Autodesk Inventor part; units mm, degrees
ref_plane "YZ Plane" through (0, 0, 0) normal (1, 0, 0) x (0, 1, 0)
ref_plane "XZ Plane" through (0, 0, 0) normal (0, 1, 0) x (-1, 0, 0)
ref_plane "XY Plane" through (0, 0, 0) normal (0, 0, 1) x (1, 0, 0)
sketch "Sketch1" plane through (0, 0, 0) normal (0, 1, 0) x (-1, 0, 0)
  line L0 (0, 0) -> (-100, 0)
  line L1 (-100, 0) -> (-100, -24.25)
  line L2 (-100, -24.25) -> (-86, -24.25)
  arc A0 (-86, -50.25) -> (-86, -24.25) centre (-86, -37.25) ccw
  line L3 (-86, -50.25) -> (-100, -50.25)
  line L4 (-100, -50.25) -> (-100, -74.5)
  line L5 (-100, -74.5) -> (0, -74.5)
  line L6 (0, -74.5) -> (0, -50.25)
  line L7 (0, -50.25) -> (-14, -50.25)
  arc A1 (-14, -24.25) -> (-14, -50.25) centre (-14, -37.25) ccw
  line L8 (-14, -24.25) -> (0, -24.25)
  line L9 (0, -24.25) -> (0, 0)
  circle A2 centre (-14, -62.25) radius 2.25
  circle A3 centre (-14, -12.25) radius 2.25
  circle A4 centre (-86, -62.25) radius 2.25
  circle A5 centre (-86, -12.25) radius 2.25
  dimension "d0" = 13
  dimension "d1" = 50
  dimension "d2" = 4.5
  dimension "d3" = 25
  dimension "d5" = 12.25
  dimension "d6" = 100
  dimension "d10" = 14
extrude "Extrusion1" add sketch "Sketch1" along normal blind 6.5
sketch "Sketch3" plane through (0, 6.5, 0) normal (0, 1, 0) x (1, 0, 0)
  line L0 (100, 74.5) -> (0, 74.5)
  line L1 (22.75, 74.5) -> (27.25, 74.5)
  line L2 (27.25, 58.2) -> (22.75, 58.2)
  line L3 (29.75, 69.5) -> (29.75, 62.2)
  line L4 (20.25, 62.2) -> (20.25, 69.5)
  line L5 (27.25, 74.5) -> (27.25, 69.5)
  line L6 (27.25, 62.2) -> (27.25, 58.2)
  line L7 (22.75, 58.2) -> (22.75, 62.2)
  line L8 (22.75, 69.5) -> (22.75, 74.5)
  line L9 (20.25, 69.5) -> (22.75, 69.5)
  line L10 (27.25, 69.5) -> (29.75, 69.5)
  line L11 (29.75, 62.2) -> (27.25, 62.2)
  line L12 (22.75, 62.2) -> (20.25, 62.2)
  line L13 (72.75, 74.5) -> (77.25, 74.5)
  line L14 (77.25, 58.2) -> (72.75, 58.2)
  line L15 (79.75, 69.5) -> (79.75, 62.2)
  line L16 (70.25, 62.2) -> (70.25, 69.5)
  line L17 (77.25, 74.5) -> (77.25, 69.5)
  line L18 (77.25, 62.2) -> (77.25, 58.2)
  line L19 (72.75, 58.2) -> (72.75, 62.2)
  line L20 (72.75, 69.5) -> (72.75, 74.5)
  line L21 (70.25, 69.5) -> (72.75, 69.5)
  line L22 (77.25, 69.5) -> (79.75, 69.5)
  line L23 (79.75, 62.2) -> (77.25, 62.2)
  line L24 (72.75, 62.2) -> (70.25, 62.2)
  line L25 (29.75, 65.85) -> (70.25, 65.85) construction
  point P0 (25, 58.2)
  point P1 (75, 58.2)
  point P2 (50, 65.85)
  point P3 (50, 74.5)
  dimension "d15" = 4.5
  dimension "d16" = 2.5
  dimension "d17" = 4
  dimension "d18" = 5
  dimension "d19" = 7.3
  dimension "d20" = 4.5
  dimension "d21" = 2.5
  dimension "d22" = 4
  dimension "d23" = 5
  dimension "d24" = 7.3
  dimension "d25" = 50
extrude "Extrusion2" cut sketch "Sketch3" against normal through all
sketch "Sketch4" plane through (0, 6.5, 0) normal (0, 1, 0) x (1, 0, 0)
  line L0 (22.75, 74.5) -> (0, 74.5)
  line L1 (100, 74.5) -> (77.25, 74.5)
  line L2 (77.25, 58.2) -> (72.75, 58.2)
  line L3 (72.75, 74.5) -> (27.25, 74.5)
  line L4 (27.25, 58.2) -> (22.75, 58.2)
  line L5 (9.5, 74.5) -> (17.5, 74.5)
  line L6 (17.5, 74.5) -> (17.5, 95.7)
  line L7 (15.5, 97.7) -> (11.5, 97.7)
  line L8 (9.5, 95.7) -> (9.5, 74.5)
  line L9 (32.5, 74.5) -> (40.5, 74.5)
  line L10 (40.5, 74.5) -> (40.5, 95.7)
  line L11 (38.5, 97.7) -> (34.5, 97.7)
  line L12 (32.5, 95.7) -> (32.5, 74.5)
  line L13 (59.5, 74.5) -> (67.5, 74.5)
  line L14 (67.5, 74.5) -> (67.5, 95.7)
  line L15 (65.5, 97.7) -> (61.5, 97.7)
  line L16 (59.5, 95.7) -> (59.5, 74.5)
  line L17 (82.5, 74.5) -> (90.5, 74.5)
  line L18 (90.5, 74.5) -> (90.5, 95.7)
  line L19 (88.5, 97.7) -> (84.5, 97.7)
  line L20 (82.5, 95.7) -> (82.5, 74.5)
  arc A0 (11.5, 97.7) -> (9.5, 95.7) centre (11.5, 95.7) ccw
  arc A1 (17.5, 95.7) -> (15.5, 97.7) centre (15.5, 95.7) ccw
  arc A2 (34.5, 97.7) -> (32.5, 95.7) centre (34.5, 95.7) ccw
  arc A3 (40.5, 95.7) -> (38.5, 97.7) centre (38.5, 95.7) ccw
  arc A4 (61.5, 97.7) -> (59.5, 95.7) centre (61.5, 95.7) ccw
  arc A5 (67.5, 95.7) -> (65.5, 97.7) centre (65.5, 95.7) ccw
  arc A6 (84.5, 97.7) -> (82.5, 95.7) centre (84.5, 95.7) ccw
  arc A7 (90.5, 95.7) -> (88.5, 97.7) centre (88.5, 95.7) ccw
  point P0 (25, 58.2)
  point P1 (75, 58.2)
  dimension "d28" = 2
  dimension "d29" = 23.2
  dimension "d30" = 8
  dimension "d31" = 8
  dimension "d32" = 8
  dimension "d33" = 8
  dimension "d34" = 15
  dimension "d35" = 15
  dimension "d36" = 7.5
  dimension "d37" = 7.5
extrude "Extrusion3" add sketch "Sketch4" against normal blind 6.5
chamfer "Chamfer1" distance 4 angle 45 2 edges at (100, 3.25, 0) (0, 3.25, 0)
chamfer "Chamfer2" distance 2 angle 45 4 edges at (100, 3.25, -24.25) (100, 3.25, -50.25) (0, 3.25, -50.25) (0, 3.25, -24.25)
sketch "Sketch5" plane through (0, 6.5, 0) normal (0, 1, 0) x (1, 0, 0)
  line L0 (4, 0) -> (96, 0)
  line L1 (34.25, 16) -> (40.75, 16)
  line L2 (40.75, 16) -> (40.75, 8)
  line L3 (40.75, 8) -> (34.25, 8)
  line L4 (34.25, 8) -> (34.25, 16)
  line L5 (59.25, 16) -> (65.75, 16)
  line L6 (65.75, 16) -> (65.75, 8)
  line L7 (65.75, 8) -> (59.25, 8)
  line L8 (59.25, 8) -> (59.25, 16)
  circle A0 centre (37.5, 23.5) radius 2.25
  circle A1 centre (62.5, 23.5) radius 2.25
  line L9 (37.5, 23.5) -> (62.5, 23.5) construction
  point P0 (0, 0)
  point P1 (37.5, 16)
  point P2 (62.5, 16)
  point P3 (50, 23.5)
  point P4 (50, 0)
  dimension "d46" = 4.5
  dimension "d47" = 6.5
  dimension "d48" = 8
  dimension "d49" = 25
  dimension "d50" = 8
  dimension "d51" = 7.5
extrude "Extrusion4" cut sketch "Sketch5" against normal through all
sketch "Sketch6" plane through (0, 6.5, 0) normal (0, 1, 0) x (1, 0, 0)
  line L0 (59.5, 74.5) -> (40.5, 74.5)
  line L1 (46.75, 40.5) -> (53.25, 40.5)
  line L2 (53.25, 40.5) -> (53.25, 32.5)
  line L3 (53.25, 32.5) -> (46.75, 32.5)
  line L4 (46.75, 32.5) -> (46.75, 40.5)
  circle A0 centre (50, 48) radius 2.25
  point P0 (0, 0)
  point P1 (50, 74.5)
  point P2 (50, 40.5)
  dimension "d54" = 6.5
  dimension "d55" = 8
  dimension "d56" = 4.5
  dimension "d57" = 7.5
  dimension "d58" = 34
extrude "Extrusion5" cut sketch "Sketch6" against normal through all
equation "\"d3\" = 0.5 * d1"
equation "\"d31\" = d30"
equation "\"d32\" = d31"
equation "\"d33\" = d32"
properties part number "x_carryage_extruder_mount"
Read the model definition and answer for the solid it produces. Units are mm, in the model's axes. A direction names the side the tool comes from. Round coordinates to 2 decimals unless told otherwise and drop trailing zeros. Write each loop counter-clockwise with the first axis right and the second up, starting at its lowest first coordinate (ties: lowest second). Pieces come first, ordered by that corner, then holes.
1. The part is cut by section C-C, the plane y = 2. State how many separate pieces and enclosed holes the cut face has, then the cut area to 3 significant figures.
2. Straight lines are drawn through the part: L1, parallel to X at y = 0.5, z = -91; L2, parallel to Z at x = 14, y = 3.25. For each, find the intervals that lie inside material, in ascending order.
3. Given pin 1 Ø2 at (y, z) = (4, -87.5) entering from -X; pin 2 Ø2.5 at (x, y) = (31, 2) entering from -Z; pin 3 Ø3 at (x, y) = (38.5, 1.5) entering from +Z; pin 4 Ø2 at (x, y) = (25, 4.5) entering from -Z, each flat-ended and moving along its own axis, determine where each tip first touches the part or whether it passes through.
4. The part is cut by section B-B, the plane z = -37.25. Determine the outline of the cut face in (x, y).
5. Which of the six approach directions +Z, -Z, +X, -X, +Y, -Y give full straight-line access (tool end or side, diameter ignored) to faces 1 (the face through (95, 3, -74.5)), 2 (the face through (30, 3, -74.5)), 3 (the face through (53.25, 3, -37))?
6. The part is cut by section D-D, the plane x = 42.5. Determine the outline of the cut face in (y, z), then the cut area to 3 significant figures.
7. Determine the mould class of faces 4 (the face through (98, 3, -2)), 5 (the face through (92, 3, -50.25)), 6 (the face through (70.25, 3, -66)) for opening direction X: pulls with the +X half, pulls with the -X half, needs draft (parallel to the pull), parting line crosses it, or undercut.
8. The part is cut by section A-A, the plane z = -78. Determine the outline of the cut face in (x, y).
Values:
1. separate pieces: 1
1. enclosed holes: 10
1. area: 6,420 mm2
2. L1: x = 9.5 to 17.5, 32.5 to 40.5, 59.5 to 67.5, 82.5 to 90.5
2. L2: z = -97.7 to -64.5, -60 to -50.25, -24.25 to -14.5, -10 to 0
3. pin 1: stops at x = 9.5
3. pin 2: stops at z = -74.5
3. pin 3: stops at z = 0
3. pin 4: stops at z = -58.2
4. outline: (27, 0) - (46.75, 0) - (46.75, 6.5) - (27, 6.5) - close; (53.25, 0) - (73, 0) - (73, 6.5) - (53.25, 6.5) - close
5. face 1: -Z, +X, +Y, -Y
5. face 2: -Z, +Y, -Y
5. face 3: +Y, -Y
6. outline: (0, -74.5) - (6.5, -74.5) - (6.5, 0) - (0, 0) - close
6. area: 484 mm2
7. face 4: pulls with the +X half
7. face 5: needs draft
7. face 6: undercut
8. outline: (9.5, 0) - (17.5, 0) - (17.5, 6.5) - (9.5, 6.5) - close; (32.5, 0) - (40.5, 0) - (40.5, 6.5) - (32.5, 6.5) - close; (59.5, 0) - (67.5, 0) - (67.5, 6.5) - (59.5, 6.5) - close; (82.5, 0) - (90.5, 0) - (90.5, 6.5) - (82.5, 6.5) - close
